```python
from build123d import *

# Parameters (mm, degrees)
RESSALTO_EXTRUS_O1_DEPTH                           = 1.5
ESBO_O2_R                                          = 17
CORTE_EXTRUS_O1_DEPTH                              = 122.865704774
FURO_ROSCADO_DE_M21_D                              = 1.6
CORTE_EXTRUS_O2_DEPTH                              = 2.5
ESCAREADO_PARA_PARAFUSO_COM_CABE_A_E_2_COUNT       = 2
ESCAREADO_PARA_PARAFUSO_COM_CABE_A_E_2_PITCH       = 7
ESCAREADO_PARA_PARAFUSO_COM_CABE_A_E_3_COUNT       = 2
ESCAREADO_PARA_PARAFUSO_COM_CABE_A_E_3_PITCH       = 41.65
ESCAREADO_PARA_PARAFUSO_COM_CABE_A_E_4_COUNT       = 2
ESCAREADO_PARA_PARAFUSO_COM_CABE_A_E_4_PITCH       = 42.234139035
ESCAREADO_PARA_PARAFUSO_COM_CABE_A_E_5_A_COUNT     = 2
ESCAREADO_PARA_PARAFUSO_COM_CABE_A_E_5_A_PITCH     = 7
ESCAREADO_PARA_PARAFUSO_COM_CABE_A_E_6_COUNT       = 2
ESCAREADO_PARA_PARAFUSO_COM_CABE_A_E_6_PITCH       = 41.65
ESCAREADO_PARA_PARAFUSO_COM_CABE_A_E_7_COUNT       = 2
ESCAREADO_PARA_PARAFUSO_COM_CABE_A_E_7_PITCH       = 42.234139035
ESCAREADO_PARA_PARAFUSO_COM_CABE_A_E_8_D           = 3.4
ESCAREADO_PARA_PARAFUSO_COM_CABE_A_E_8_DEPTH       = 7.25
ESCAREADO_PARA_PARAFUSO_COM_CABE_A_E_8_CSINK_D     = 6.3
ESCAREADO_PARA_PARAFUSO_COM_CABE_A_E_8_CSINK_ANGLE = 90
ESCAREADO_PARA_PARAFUSO_COM_CABE_A_E_8_TIP         = 1.021463052
CORTE_EXTRUS_O3_DEPTH                              = 122.865704775
CORTE_EXTRUS_O4_DEPTH                              = 122.865704775
CORTE_EXTRUS_O5_DEPTH                              = 115.773877222
CORTE_EXTRUS_O6_DEPTH                              = 112.164853797
FILETE2_R                                          = 2
BROCA_DE_ROSQUEAR_PARA_TARRAXA_DE_M31_D            = 2.5


with BuildPart() as part:
    # Esboço1 → Ressalto-extrusão1 (new body)
    with BuildSketch(Plane(origin=(0, 0, 0), x_dir=(1, 0, 0), z_dir=(0, 1, 0))):
        with BuildLine():
            Line((17, -85.322916031), (17, 85.322916031))
            ThreePointArc((17, 85.322916031), (87, 0), (17, -85.322916031))
        make_face()
    extrude(amount=RESSALTO_EXTRUS_O1_DEPTH)

    # Esboço2 → Corte-extrusão1 (cut, through all)
    with BuildSketch(Plane(origin=(0, 1.5, 0), x_dir=(1, 0, 0), z_dir=(0, 1, 0))):
        with Locations(Location((61, 0, 0), (0, 0, 270))):
            Circle(ESBO_O2_R)
    extrude(amount=-CORTE_EXTRUS_O1_DEPTH, mode=Mode.SUBTRACT)

    # Furo roscado de M21 (through all)
    with Locations(Plane(origin=(71, 1.5, 17.320508076), x_dir=(0, 0, 1), z_dir=(0, 1, 0))):
        with Locations((0, 0), (-17.320508076, -30), (-34.641016152, 0)):
            Hole(FURO_ROSCADO_DE_M21_D / 2)

    # Esboço4 → Corte-extrusão2 (cut)
    with BuildSketch(Plane(origin=(0, 1.5, 0), x_dir=(1, 0, 0), z_dir=(0, 1, 0))):
        with BuildLine():
            Line((30, 0), (30, 24.445048467))
            ThreePointArc((30, 24.445048467), (29.879385242, 25.129088753), (29.532088886, 25.730623686))
            Line((29.532088886, 25.730623686), (17, 40.665785639))
            Line((17, 40.665785639), (17, -40.665785639))
            Line((17, -40.665785639), (29.532088886, -25.730623686))
            ThreePointArc((29.532088886, -25.730623686), (29.879385242, -25.129088753), (30, -24.445048467))
            Line((30, -24.445048467), (30, 0))
        make_face()
    extrude(amount=-CORTE_EXTRUS_O2_DEPTH, mode=Mode.SUBTRACT)

    # Esboço6 → Escareado para parafuso com cabe_a escar (revolve, cut)
    with BuildSketch(Plane(origin=(33.786228885, 1.5, -55.535118997), x_dir=(0, 0, 1), z_dir=(1, 0, 0))):
        Polygon((0, 0), (0, 1.5), (1.7, 1.5), (1.7, 1.45), (3.15, 0), align=None)
    escareado_para_parafuso_com_cabe_a_escar = revolve(axis=Axis((33.786228885, 7.85, -55.535118997), (0, -1, 0)), mode=Mode.SUBTRACT)

    # Escareado para parafuso com cabe_a e 2: Escareado para parafuso com cabe_a escar ×2
    with Locations(*[Vector(-0.7660444431189771, 0, 0.6427876096865406) * (i * ESCAREADO_PARA_PARAFUSO_COM_CABE_A_E_2_PITCH) for i in range(1, ESCAREADO_PARA_PARAFUSO_COM_CABE_A_E_2_COUNT)]):
        add(escareado_para_parafuso_com_cabe_a_escar, mode=Mode.SUBTRACT)

    # Escareado para parafuso com cabe_a e 3: Escareado para parafuso com cabe_a escar ×2
    with Locations(*[Vector(0.642787609686541, 0, 0.7660444431189767) * (i * ESCAREADO_PARA_PARAFUSO_COM_CABE_A_E_3_PITCH) for i in range(1, ESCAREADO_PARA_PARAFUSO_COM_CABE_A_E_3_COUNT)]):
        add(escareado_para_parafuso_com_cabe_a_escar, mode=Mode.SUBTRACT)

    # Escareado para parafuso com cabe_a e 4: Escareado para parafuso com cabe_a escar ×2
    with Locations(*[Vector(0.5069309646406032, 0, 0.8619866571406704) * (i * ESCAREADO_PARA_PARAFUSO_COM_CABE_A_E_4_PITCH) for i in range(1, ESCAREADO_PARA_PARAFUSO_COM_CABE_A_E_4_COUNT)]):
        add(escareado_para_parafuso_com_cabe_a_escar, mode=Mode.SUBTRACT)

    # Esboço7 → Escareado para parafuso com cabe_a e 5 (revolve, cut)
    with BuildSketch(Plane(origin=(55.196021727, 1.5, 19.129854673), x_dir=(0, 0, 1), z_dir=(1, 0, 0))):
        Polygon((0, 0), (0, 1.5), (1.7, 1.5), (1.7, 1.45), (3.15, 0), align=None)
    escareado_para_parafuso_com_cabe_a_e_5 = revolve(axis=Axis((55.196021727, 7.85, 19.129854673), (0, -1, 0)), mode=Mode.SUBTRACT)

    # Escareado para parafuso com cabe_a e 5 a: Escareado para parafuso com cabe_a e 5 ×2
    with Locations(*[Vector(0.7660444431189781, 0, 0.6427876096865394) * (i * ESCAREADO_PARA_PARAFUSO_COM_CABE_A_E_5_A_PITCH) for i in range(1, ESCAREADO_PARA_PARAFUSO_COM_CABE_A_E_5_A_COUNT)]):
        add(escareado_para_parafuso_com_cabe_a_e_5, mode=Mode.SUBTRACT)

    # Escareado para parafuso com cabe_a e 6: Escareado para parafuso com cabe_a e 5 ×2
    with Locations(*[Vector(-0.64278760968654, 0, 0.7660444431189776) * (i * ESCAREADO_PARA_PARAFUSO_COM_CABE_A_E_6_PITCH) for i in range(1, ESCAREADO_PARA_PARAFUSO_COM_CABE_A_E_6_COUNT)]):
        add(escareado_para_parafuso_com_cabe_a_e_5, mode=Mode.SUBTRACT)

    # Escareado para parafuso com cabe_a e 7: Escareado para parafuso com cabe_a e 5 ×2
    with Locations(*[Vector(-0.5069309646406018, 0, 0.8619866571406711) * (i * ESCAREADO_PARA_PARAFUSO_COM_CABE_A_E_7_PITCH) for i in range(1, ESCAREADO_PARA_PARAFUSO_COM_CABE_A_E_7_COUNT)]):
        add(escareado_para_parafuso_com_cabe_a_e_5, mode=Mode.SUBTRACT)

    # Escareado para parafuso com cabe_a e 8
    with Locations(Plane(origin=(48.209070726, 0, 57.453333234), x_dir=(0, 0, -1), z_dir=(0, -1, 0))):
        with Locations((0, 0), (19.953333234, 16.742834558), (94.953333234, 16.742834558), (110.486341823, 4.823937863)):
            CounterSinkHole(ESCAREADO_PARA_PARAFUSO_COM_CABE_A_E_8_D / 2, ESCAREADO_PARA_PARAFUSO_COM_CABE_A_E_8_CSINK_D / 2, depth=ESCAREADO_PARA_PARAFUSO_COM_CABE_A_E_8_DEPTH, counter_sink_angle=ESCAREADO_PARA_PARAFUSO_COM_CABE_A_E_8_CSINK_ANGLE)
            with Locations((0, 0, -(ESCAREADO_PARA_PARAFUSO_COM_CABE_A_E_8_DEPTH + ESCAREADO_PARA_PARAFUSO_COM_CABE_A_E_8_TIP / 2))):  # 118° drill point
                Cone(0, ESCAREADO_PARA_PARAFUSO_COM_CABE_A_E_8_D / 2, ESCAREADO_PARA_PARAFUSO_COM_CABE_A_E_8_TIP, mode=Mode.SUBTRACT)

    # Esboço17 → Corte-extrusão3 (cut, through all)
    with BuildSketch(Plane.XZ):
        Polygon((26.495554955, -53.333739059), (17, -45.366022398), (17, -85.322916031), (48.78373029, -85.322916031), (48.78373029, -72.035738762), align=None)
    extrude(amount=-CORTE_EXTRUS_O3_DEPTH, mode=Mode.SUBTRACT)

    # Esboço18 → Corte-extrusão4 (cut, through all)
    with BuildSketch(Plane(origin=(0, 1.5, 0), x_dir=(1, 0, 0), z_dir=(0, 1, 0))):
        Polygon((23.281616906, -57.163961274), (17, -51.893058845), (17, -85.322916031), (56.840152401, -85.322916031), align=None)
    extrude(amount=-CORTE_EXTRUS_O4_DEPTH, mode=Mode.SUBTRACT)

    # Esboço19 → Corte-extrusão5 (cut, through all)
    with BuildSketch(Plane(origin=(0, 1.5, 0), x_dir=(1, 0, 0), z_dir=(0, 1, 0))):
        with BuildLine():
            Line((48.78373029, 72.035738762), (46.390783088, 70.027817648))
            ThreePointArc((46.390783088, 70.027817648), (83.958731282, -2.632763095), (41.91211377, -72.796804321))
            Line((41.91211377, -72.796804321), (44.35320854, -74.845126042))
            ThreePointArc((44.35320854, -74.845126042), (86.960447647, -2.623079291), (48.78373029, 72.035738762))
        make_face()
    extrude(amount=-CORTE_EXTRUS_O5_DEPTH, mode=Mode.SUBTRACT)

    # Esboço20 → Corte-extrusão6 (cut, through all)
    with BuildSketch(Plane(origin=(0, 1.5, 0), x_dir=(1, 0, 0), z_dir=(0, 1, 0))):
        Polygon((41.028471986, 65.52830438), (42.314047206, 63.996215494), (48.108978901, 68.858740542), (46.823403682, 70.390829428), align=None)
    extrude(amount=-CORTE_EXTRUS_O6_DEPTH, mode=Mode.SUBTRACT)

    # Filete2
    filete2_edges = [part.edges().sort_by_distance(p)[0] for p in [
        (17, 0.75, 40.665785639),
        (17, 0.75, 51.893058845),
        (41.91211377, 0.75, 72.796804321),
        (48.108978901, 0.75, -68.858740542),
        (41.028471986, 0.75, -65.52830438),
        (17, 0.75, -40.665785639),
        (17, 0.75, -45.366022398),
    ]]
    fillet(filete2_edges, radius=FILETE2_R - 0.0001)  # a hair under: the kernel refuses the full size

    # Broca de rosquear para tarraxa de M31 (through all)
    with Locations(Plane(origin=(30, 1.5, 44), x_dir=(0, 0, 1), z_dir=(0, 1, 0))):
        with Locations((0, 0), (-8, 0), (-88, 0), (-80, 0)):
            Hole(BROCA_DE_ROSQUEAR_PARA_TARRAXA_DE_M31_D / 2)


solid = part.part
```
The model under review builds one solid part; all positions refer to its coordinate system, in mm. A direction names the side the tool comes from. Coordinates: 2 decimals unless noted, no trailing zeros. Write each loop counter-clockwise with the first axis right and the second up, starting at its lowest first coordinate (ties: lowest second). Pieces come first, ordered by that corner, then holes. Notation, with made-up numbers: (-5, 6.25) -> (7, 6.25) arc R13 ccw to (7, 16.25) -> close; hole circle Ø10 at (30.5, -32). An arc over 180 degrees is marked (long way). One line per item, written item: value. Start each with the question number.
Q1. The part is to be moulded in two halves that separate along Z. For faces 3 (the face through (83.96, 0.76, 2.58)), 4 (the face through (30.05, 0.74, 45.25)), 5 (the face through (43.5, 0, 1)), say which applies: +Z half, -Z half, draft (parallel to the pull), parting line (faces both ways), or undercut.
Q2. Add section A-A, the plane z = 13. Give the boundary of the cut face in (x, y).
Q3. For faces 1 (the face through (23.416, 0.76, 33.02)), 2 (the face through (44.586, 0.76, -65.903)), list the 3-axis set-ups (+Z, -Z, +X, -X, +Y, -Y) from which the entire face can be reached by the end or side of a thin tool; tool diameter is ignored.
Q4. To check wall thickness, follow probe 1 along Z at (x, y) = (62.5, 1.45); probe 2 along X at (y, z) = (0.7, -18); probe 3 along X at (y, z) = (0.6, 1). State the ranges of each line that lie inside material, in increasing order.
Q5. Clearance check with flat-ended pins moving along their axes: P1, Ø3, axis at x = 55.2, z = -19.13, coming from the -Y side; P2, Ø4.5, axis at x = 60.56, z = 23.63, coming from the +Y side; P3, Ø4, axis at x = 55.2, z = 19.13, coming from the +Y side; P4, Ø4.5, axis at x = 64.95, z = 37.5, coming from the -Y side. State where each tip first meets the part, or that it passes through.
Q6. Add section B-B, the plane z = 44. Give the boundary of the cut face in (x, y), then the cut area to 3 significant figures.
Response:
1. face 3: parting line
1. face 4: undercut
1. face 5: draft
2. outline: (30, 0) -> (50.05, 0) -> (50.05, 1.5) -> (30, 1.5) -> close; (71.95, 0) -> (82.99, 0) -> (82.99, 1.5) -> (71.95, 1.5) -> close
3. face 1: -X, +Y, -Y
3. face 2: -Z, +Y, -Y
4. probe 1: -56.12 to -26.05, -21.21 to -16.93, 16.93 to 21.21, 26.05 to 56.12
4. probe 2: 30 to 53.14, 57.26 to 70.58, 71.42 to 82.05
4. probe 3: 30 to 44.03, 77.97 to 83.99
5. P1: through
5. P2: y = 0.6
5. P3: y = 0.35
5. P4: y = 0.9
6. outline: (17, 0) -> (28.75, 0) -> (28.75, 1.5) -> (17, 1.5) -> close; (31.25, 0) -> (71.55, 0) -> (71.55, 1.5) -> (31.25, 1.5) -> close
6. area: 78.1 mm²
